Work out the finished part from the listing and answer in its coordinate system (mm). A direction names the side the tool comes from. Round coordinates to 2 decimals unless told otherwise and drop trailing zeros. Write each loop counter-clockwise with the first axis right and the second up, starting at its lowest first coordinate (ties: lowest second). Pieces come first, ordered by that corner, then holes.
1. Flat-ended cylindrical pins translate along their axes: pin 1 Ø12 at (x, y) = (8.5, 28.5) entering from -Z; pin 2 Ø8 at (y, z) = (55, -7) entering from -X; pin 3 Ø9 at (x, y) = (3, 141.5) entering from -Z; pin 4 Ø5 at (x, y) = (0, 213) entering from -Z. Find the tip coordinate at first contact, or state that the pin passes through.
2. Determine the mould class of faces 1 (the face through (-12.5, 250.38, -6.46)), 2 (the face through (12.46, 215.6, -14.61)), 3 (the face through (0, -8, 0)), 4 (the face through (-10.21, 210.46, -20.95)) for opening direction Y: pulls with the +Y half, pulls with the -Y half, needs draft (parallel to the pull), parting line crosses it, or undercut.
3. Straight lines are drawn through the part: probe 1 along X at (y, z) = (213, 6.95); probe 2 along Z at (x, y) = (7, 212); probe 3 along Z at (x, y) = (2, 194.5). For each, find the intervals that lie inside material, in ascending order.
4. Find section B-B (x = -0.5). Count the separate pieces of the cut face and the enclosed holes in it, and give its area (3 significant figures).
5. A tool of negligible diameter and unlimited length cuts with its end or side. For faces 5 (the face through (0, 140, 3)), 6 (the face through (10, 225, -12)), 7 (the face through (0, 195.144, -21)), from which of +Z, -Z, +X, -X, +Y, -Y can it reach the whole face along a straight path? Write none if from no direction.
6. Find section A-A (y = 257). Write down the section's boundary in (x, z).
```python
from build123d import *

# Parameters (mm, degrees)
BOSS_EXTRUDE1_DEPTH      = 15
BOSS_EXTRUDE1_DEPTH_BACK = 15
SKETCH1_R                = 4.05
SKETCH1_R_2              = 15.1
CUT_EXTRUDE2_DEPTH       = 10
CUT_EXTRUDE2_DEPTH_BACK  = 10
SKETCH5_W                = 66.834238055
SKETCH5_H                = 69.856255641
CUT_EXTRUDE1_DEPTH       = 274.313007374
CUT_EXTRUDE1_DEPTH_BACK  = 274.313007374
FILLET1_R                = 3
FILLET2_R                = 5
SKETCH6_R                = 3
CUT_EXTRUDE3_DEPTH       = 5


with BuildPart() as part:
    # Sketch1 → Boss-Extrude1 (new, two sides: drawn at the far end of the back side and taken through both)
    with BuildSketch(Plane(origin=(0, 0, 0), x_dir=(0, 0, -1), z_dir=(1, 0, 0)).offset(-BOSS_EXTRUDE1_DEPTH_BACK)):
        with BuildLine():
            Line((-8, 0), (-8, 270))
            Line((-8, 270), (7, 270))
            Line((7, 270), (29.498971947, 173.978261275))
            ThreePointArc((29.498971947, 173.978261275), (29.975942027, 170.599581269), (29.840899654, 167.190073592))
            Line((29.840899654, 167.190073592), (7.933010381, -1.033124533))
            ThreePointArc((7.933010381, -1.033124533), (-0.517647059, -7.983235029), (-8, 0))
        make_face()
        Circle(SKETCH1_R, mode=Mode.SUBTRACT)
        with Locations((11, 169.643744359)):
            Circle(SKETCH1_R_2, mode=Mode.SUBTRACT)
    extrude(amount=BOSS_EXTRUDE1_DEPTH + BOSS_EXTRUDE1_DEPTH_BACK)

    # Sketch5 → Cut-Extrude2 (cut, two sides: drawn at the far end of the back side and taken through both)
    with BuildSketch(Plane(origin=(0, 0, 0), x_dir=(0, 0, -1), z_dir=(1, 0, 0)).offset(-CUT_EXTRUDE2_DEPTH_BACK)):
        with Locations((30.417119028, 230.07187218)):
            Rectangle(SKETCH5_W, SKETCH5_H)
    extrude(amount=CUT_EXTRUDE2_DEPTH + CUT_EXTRUDE2_DEPTH_BACK, mode=Mode.SUBTRACT)

    # Sketch4 → Cut-Extrude1 (cut, two sides: drawn at the far end of the back side and taken through both)
    with BuildSketch(Plane(origin=(15, 0, 0), x_dir=(0, 0, -1), z_dir=(1, 0, 0)).offset(-CUT_EXTRUDE1_DEPTH_BACK)):
        with BuildLine():
            ThreePointArc((23.038271938, 153.672519962), (9.705882353, 149.685656787), (-3, 155.360887501))
            Line((-3, 155.360887501), (-3, 130.360887501))
            Line((-3, 130.360887501), (15.768762187, 97.852437799))
            Line((15.768762187, 97.852437799), (23.038271938, 153.672519962))
        make_face()
        with BuildLine():
            Line((-3, 208.232171682), (-3, 183.926601216))
            ThreePointArc((-3, 183.926601216), (8.703485357, 189.511457375), (21.372438031, 186.743818314))
            Line((21.372438031, 186.743818314), (19.626242772, 194.196279044))
            Line((19.626242772, 194.196279044), (-3, 208.232171682))
        make_face()
        Polygon((14.706143018, 89.692948188), (-3, 120.360887501), (-3, 59.025008875), align=None)
        Polygon((-3, 234.116085841), (-3, 214.116085841), (18.013102612, 201.080883522), (12.529881351, 224.48232784), align=None)
        with BuildLine():
            Line((13.024511965, 76.780277764), (-3, 49.025008875))
            Line((-3, 49.025008875), (-3, 8.485281374))
            ThreePointArc((-3, 8.485281374), (0.582352941, 8.981139407), (4.070672938, 8.026806453))
            Line((4.070672938, 8.026806453), (13.024511965, 76.780277764))
        make_face()
        Polygon((-3, 265), (-3, 240), (10.916741191, 231.366932319), (3.03613565, 265), align=None)
    extrude(amount=CUT_EXTRUDE1_DEPTH + CUT_EXTRUDE1_DEPTH_BACK, mode=Mode.SUBTRACT)

    # Fillet1
    fillet1_edges = [part.edges().sort_by_distance(p)[0] for p in [
        (0, 89.692948188, -14.706143018),
        (0, 59.025008875, 3),
        (0, 120.360887501, 3),
        (12.5, 240, 3),
        (12.5, 265, -3.03613565),
        (12.5, 231.366932319, -10.916741191),
        (-12.5, 240, 3),
        (-12.5, 265, -3.03613565),
        (-12.5, 231.366932319, -10.916741191),
        (0, 183.926601216, 3),
        (12.5, 208.232171682, 3),
        (-12.5, 208.232171682, 3),
        (0, 186.743818314, -21.372438031),
        (0, 194.196279044, -19.626242772),
        (0, 8.026806453, -4.070672938),
        (0, 8.485281374, 3),
        (0, 49.025008875, 3),
        (0, 76.780277764, -13.024511965),
        (12.5, 214.116085841, 3),
        (12.5, 234.116085841, 3),
        (12.5, 224.48232784, -12.529881351),
        (12.5, 201.080883522, -18.013102612),
        (-12.5, 214.116085841, 3),
        (-12.5, 234.116085841, 3),
        (-12.5, 224.48232784, -12.529881351),
        (-12.5, 201.080883522, -18.013102612),
        (0, 155.360887501, 3),
        (0, 153.672519962, -23.038271938),
        (0, 97.852437799, -15.768762187),
        (0, 130.360887501, 3),
        (0, 265, 3),
        (-10, 265, -5.603845906),
        (10, 265, -5.603845906),
        (-10, 195.143744359, -21.319282147),
        (10, 195.143744359, -21.319282147),
    ]]
    fillet(fillet1_edges, radius=FILLET1_R)

    # Fillet2
    fillet2_edges = [part.edges().sort_by_distance(p)[0] for p in [
        (0, 270, 8),
        (0, 270, -7),
    ]]
    fillet(fillet2_edges, radius=FILLET2_R)

    # Sketch6 → Cut-Extrude3 (cut)
    with BuildSketch(Plane.XY.offset(8)):
        with Locations((0, 257)):
            Circle(SKETCH6_R)
        with Locations((0, 213)):
            Circle(SKETCH6_R)
    extrude(amount=-CUT_EXTRUDE3_DEPTH, mode=Mode.SUBTRACT)


solid = part.part
```
Worked answers:
1. pin 1: stops at z = -12.56
1. pin 2: stops at x = -15
1. pin 3: stops at z = -27.08
1. pin 4: passes through
2. face 1: undercut
2. face 2: undercut
2. face 3: pulls with the -Y half
2. face 4: pulls with the +Y half
3. probe 1: x = -15 to -3, 3 to 15
3. probe 2: z = 3 to 8
3. probe 3: z = -24.69 to -19.03, 3 to 8
4. separate pieces: 3
4. enclosed holes: 5
4. area: 3,170 mm2
5. face 5: +X, -X
5. face 6: -Z
5. face 7: -Z, +Y
6. outline: (-15, -10.05) - (-10, -10.05) - (-10, -4.91) - (-15, -4.91) - close; (-15, 3) - (-3, 3) - (-3, 8) - (-15, 8) - close; (3, 3) - (15, 3) - (15, 8) - (3, 8) - close; (10, -10.05) - (15, -10.05) - (15, -4.91) - (10, -4.91) - close
